Build history of the part. All positions in model axes, mm. Face numbers are marked on the shaded views. A direction names the side the tool comes from. Round coordinates to 2 decimals unless told otherwise and drop trailing zeros. Order: outer loops, then holes, each group sorted by start corner. A loop starts at its lowest first (then second) coordinate and runs counter-clockwise, first axis right, second up. Notation, with made-up numbers: (-8.5, 60) - (49.5, 60) arc R34 ccw to (49.5, 91) - close; hole circle Ø9 at (-5.5, 32). An arc over 180 degrees is marked (long way). One line per question, with ' | ' between items. Start each with the question number.
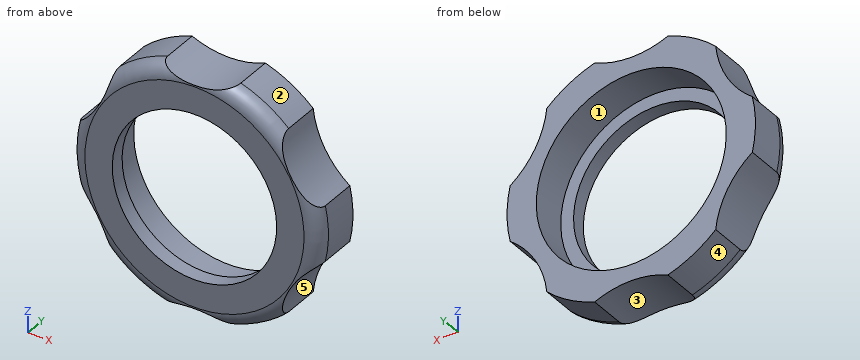
Autodesk Inventor part; units mm, degrees
ref_plane "YZ Plane" through (0, 0, 0) normal (1, 0, 0) x (0, 1, 0)
ref_plane "XZ Plane" through (0, 0, 0) normal (0, 1, 0) x (-1, 0, 0)
ref_plane "XY Plane" through (0, 0, 0) normal (0, 0, 1) x (1, 0, 0)
sketch "Эскиз1" plane through (0, 0, 0) normal (1, 0, 0) x (0, 1, 0)
  line L0 (0, 0) -> (0, 30)
  line L1 (0, 0) -> (4, 0)
  line L2 (4, 0) -> (4, 26)
  line L3 (4, 26) -> (14, 26)
  line L4 (14, 26) -> (14, 34)
  line L5 (14, 34) -> (4, 34)
  arc A0 (4, 34) -> (0, 30) centre (4, 30) ccw
  point P0 (0, 30)
  dimension "d2" = 4
revolve "Вращение1" add sketch "Эскиз1" angle 360 about axis through (0, 0, 0) along (0, 1, 0)
sketch "Эскиз2" plane through (0, 0, 0) normal (0, -1, 0) x (1, 0, 0)
  circle A0 centre (0, 0) radius 30
sketch "Эскиз3" plane through (0, 0, 0) normal (0, -1, 0) x (1, 0, 0)
  circle A0 centre (0, 0) radius 30
  circle A1 centre (0, 0) radius 30
hole "Отверстие1" at (0, 0, 0) direction (0, 1, 0) diameter 45 end through all
sketch "Эскиз4" plane through (0, 0, 0) normal (0, -1, 0) x (1, 0, 0)
  circle A0 centre (0, 0) radius 30
  circle A1 centre (0, 55.1977) radius 24.8245
  circle A2 centre (47.8026, 27.5988) radius 24.8245
  circle A3 centre (47.8026, -27.5988) radius 24.8245
  circle A4 centre (0, -55.1977) radius 24.8245
  circle A5 centre (-47.8026, -27.5988) radius 24.8245
  circle A6 centre (-47.8026, 27.5988) radius 24.8245
  dimension "d18" = 360
extrude "Выдавливание1" cut sketch "Эскиз4" along normal through all both and the other way through all contours A1 | A2 | A3 | A4 | A5 | A6
thread "Резьба1"
properties part number "Крышка"
Item 1: Slice it at D-D (y = 2.25). Write the cut outline in (x, z), plus the area to 3 significant figures.
Item 2: Pin check, flat tips, straight feed: pin 1 (3 mm diameter, centred on y = 5, z = -20.5, fed in from -X); pin 2 (1.5 mm diameter, centred on x = -7, y = 2, fed in from -Z); pin 3 (3 mm diameter, centred on y = 8.5, z = 15.5, fed in from -X); pin 4 (4 mm diameter, centred on x = 12, y = 11.5, fed in from +Z). Stop position of each tip, or through.
Item 3: Wall check: line 1 along X through (y, z) = (7.25, 0); line 2 along Z through (x, y) = (0, 2.65); line 3 along X through (y, z) = (1.25, -17). Give the ranges that are in metal, low to high. Write a range as [from, to].
Item 4: Slice it at B-B (x = 0). Write the cut outline in (y, z).
Item 5: Slice it at A-A (z = 0). Write the cut outline in (x, y), plus the area to 3 significant figures.
Item 6: Pull direction X, two halves, no side cores. Call the marked faces 3, 4 and 5: released by +X, released by -X, zero draft, split by the parting line, or undercut.
Item 7: Slice it at C-C (y = 8.5). Write the cut outline in (x, z).
Item 8: 3-axis set-ups, long thin cutter, end or side, ignore diameter. For the marked faces 1 and 2: which of +Z, -Z, +X, -X, +Y, -Y reach the whole face in a straight line?
A:
1) outline: (-32.65, -7.94) arc R24.82 cw to (-23.2, -24.3) arc R33.6 ccw to (-9.45, -32.24) arc R24.82 cw to (9.45, -32.24) arc R33.6 ccw to (23.2, -24.3) arc R24.82 cw to (32.65, -7.94) arc R33.6 ccw to (32.65, 7.94) arc R24.82 cw to (23.2, 24.3) arc R33.6 ccw to (9.45, 32.24) arc R24.82 cw to (-9.45, 32.24) arc R33.6 ccw to (-23.2, 24.3) arc R24.82 cw to (-32.65, 7.94) arc R33.6 ccw to start; hole circle Ø45 at (0, 0) | area: 1,710 mm^2
2) pin 1: x = -24.51 | pin 2: z = -31.61 | pin 3: x = -27.03 | pin 4: z = 32.49
3) line 1: [-34, -26], [26, 34] | line 2: [-30.37, -22.5], [22.5, 30.37] | line 3: [-25.35, -14.74], [14.74, 25.35]
4) outline: (0, -30) arc R4 ccw to (0.02, -30.37) - (14, -30.37) - (14, -26) - (4, -26) - (4, -22.5) - (0, -22.5) - close; (0, 22.5) - (4, 22.5) - (4, 26) - (14, 26) - (14, 30.37) - (0.02, 30.37) arc R4 ccw to (0, 30) - close
5) outline: (-34, 4) arc R4 ccw to (-30, 0) - (-22.5, 0) - (-22.5, 4) - (-26, 4) - (-26, 14) - (-34, 14) - close; (22.5, 0) - (30, 0) arc R4 ccw to (34, 4) - (34, 14) - (26, 14) - (26, 4) - (22.5, 4) - close | area: 245 mm^2
6) face 3: undercut | face 4: released by -X | face 5: released by +X
7) outline: (-33.15, -7.56) arc R24.82 cw to (-23.12, -24.93) arc R34 ccw to (-10.03, -32.49) arc R24.82 cw to (10.03, -32.49) arc R34 ccw to (23.12, -24.93) arc R24.82 cw to (33.15, -7.56) arc R34 ccw to (33.15, 7.56) arc R24.82 cw to (23.12, 24.93) arc R34 ccw to (10.03, 32.49) arc R24.82 cw to (-10.03, 32.49) arc R34 ccw to (-23.12, 24.93) arc R24.82 cw to (-33.15, 7.56) arc R34 ccw to start; hole circle Ø52 at (0, 0)
8) face 1: +Y | face 2: +Z, +X, +Y, -Y
